Source: CAD feature listing. Evaluate the final solid. Frame: model axes, mm. A direction names the side the tool comes from. Round coordinates to 2 decimals unless told otherwise and drop trailing zeros. Order: outer loops, then holes, each group sorted by start corner. A loop starts at its lowest first (then second) coordinate and runs counter-clockwise, first axis right, second up. Notation, with made-up numbers: (48, 18.5) - (104, 18.5) arc R10 ccw to (104, 37.5) - close; hole circle Ø1 at (17.25, 70). An arc over 180 degrees is marked (long way). Return JSON: item names as keys, results as strings. Group by question number.
1) Section C-C, the plane x = 23. Return loops of the section in (y, z) (3 decimals), plus the area to 3 significant figures.
2) Section B-B, the plane y = -2.25. Return loops of the section in (x, z).
3) Access query for faces 1 (the flat face through (23, -2, 115.698)), 2 (the flat face through (29.383, -2, 224)), 3 (the flat face through (16.683, -2, 224)). Directions: +Z, -Z, +X, -X, +Y, -Y. A direction counts if a zero-diameter tool reaches every point of the face in a straight line with its end or side. Return the directions, or none.
4) Ray query, line 1 (X direction, y = -3.45, z = 115.5); line 2 (Z direction, x = -39.5, y = -2.5); line 3 (X direction, y = -1.6, z = 196.5). Return the intervals inside material, ascending. Write a range as from..to.
5) Section A-A, the plane z = 194.5. Return loops of the section in (x, y) (3 decimals), plus the area to 3 significant figures.
6) Section D-D, the plane z = 113.5. Return loops of the section in (x, y) (3 decimals).
7) Mould query, pull axis X, two halves, no side actions, for faces 4 (the flat face through (-43.642, -2, 161)), 5 (the cylindrical face through (-8.282, -2.191, 191.777)), 6 (the flat face through (31, -2, 217.298)). Classes: pulls with the +X half, pulls with the -X half, needs draft (parallel to the pull), parting line crosses it, or undercut.
8) Contact query for a flat-ended pin moving along its axis: P1, Ø1.3, axis at x = -38, y = -3, coming from the +Z side. Output: stop coordinate, or through.
```python
from build123d import *

# Parameters (mm, degrees)
F1_DEPTH = 4.445


with BuildPart() as f1:
    # F0 (on Front) → F1 (new body)
    with BuildSketch(Plane.XZ):
        with BuildLine():
            Line((-34.370821, 217.297887), (-43.641821, 217.297887))
            Line((-43.641821, 217.297887), (-43.641821, 102.997887))
            Line((-43.641821, 102.997887), (16.683179, 102.997887))
            Line((16.683179, 102.997887), (16.683179, 115.697887))
            Line((16.683179, 115.697887), (28.589429, 115.697887))
            Line((28.589429, 115.697887), (28.589429, 102.997887))
            Line((28.589429, 102.997887), (29.383179, 102.997887))
            Line((29.383179, 102.997887), (32.558179, 102.997887))
            Line((32.558179, 102.997887), (32.558179, 217.297887))
            Line((32.558179, 217.297887), (29.383179, 217.297887))
            Line((29.383179, 217.297887), (29.383179, 229.997887))
            Line((29.383179, 229.997887), (16.683179, 229.997887))
            Line((16.683179, 229.997887), (16.683179, 217.297887))
            ThreePointArc((16.683179, 217.297887), (-8.843821, 191.770887), (-34.370821, 217.297887))
        make_face()
    extrude(amount=F1_DEPTH)


solid = f1.part
```
Geometry check:
{
 "1": {"outline": "(-4.445, 115.698) - (0, 115.698) - (0, 229.998) - (-4.445, 229.998) - close", "area": "508 mm2"},
 "2": {"outline": "(-43.64, 103) - (16.68, 103) - (16.68, 115.7) - (28.59, 115.7) - (28.59, 103) - (32.56, 103) - (32.56, 217.3) - (29.38, 217.3) - (29.38, 230) - (16.68, 230) - (16.68, 217.3) arc R25.53 cw to (-34.37, 217.3) - (-43.64, 217.3) - close"},
 "3": {"face 1": "-Z, +Y, -Y", "face 2": "+Z, +X, +Y, -Y", "face 3": "+Z, -X, +Y, -Y"},
 "4": {"line 1": "-43.64..16.68, 28.59..32.56", "line 2": "103..217.3", "line 3": "-43.64..-23.65, 5.96..32.56"},
 "5": {"outline": "(-43.642, -4.445) - (-20.328, -4.445) - (-20.328, 0) - (-43.642, 0) - close; (2.64, -4.445) - (32.558, -4.445) - (32.558, 0) - (2.64, 0) - close", "area": "237 mm2"},
 "6": {"outline": "(-43.642, -4.445) - (16.683, -4.445) - (16.683, 0) - (-43.642, 0) - close; (28.589, -4.445) - (32.558, -4.445) - (32.558, 0) - (28.589, 0) - close"},
 "7": {"face 4": "pulls with the -X half", "face 5": "undercut", "face 6": "needs draft"},
 "8": {"P1": "z = 217.3"}
}
